from build123d import *

# Parameters (mm, degrees)
F1_DEPTH = 63.5
F0_W     = 19.703557321
F0_H     = 14.5021951942
F2_DEPTH = 25.4
F3_DEPTH = 7.9375
F5_R     = 6.35


with BuildPart() as f1:
    # F0 (on Front) → F1 (new body, symmetric)
    with BuildSketch(Plane.XZ):
        Polygon((-41.275, 9.525), (-41.275, -9.525), (41.275, -9.525), (41.275, 9.525), (22.225, 9.525), align=None)
    extrude(amount=F1_DEPTH, both=True)

    # F0 (on Front) → F2 (join, symmetric)
    with BuildSketch(Plane.XZ):
        with BuildLine():
            Line((22.225, 9.525), (41.275, 9.525))
            Line((41.275, 9.525), (41.275, 31.7500035657))
            ThreePointArc((41.275, 31.7500035657), (44.6674064176, 39.9399971481), (52.8574, 43.3324035657))
            Line((52.8574, 43.3324035657), (64.774647217, 43.3324035657))
            Line((64.774647217, 43.3324035657), (64.774647217, 57.8345987598))
            Line((64.774647217, 57.8345987598), (84.478204538, 57.8345987598))
            Line((84.478204538, 57.8345987598), (84.478204538, 62.3824035657))
            Line((84.478204538, 62.3824035657), (52.8574, 62.3824035657))
            ThreePointArc((52.8574, 62.3824035657), (31.197022236, 53.4103813297), (22.225, 31.7500035657))
            Line((22.225, 31.7500035657), (22.225, 9.525))
        make_face()
        with Locations((74.6264258775, 50.5835011627)):
            Rectangle(F0_W, F0_H)
    extrude(amount=F2_DEPTH, both=True)

    # F0 (on Front) → F3 (join, symmetric)
    with BuildSketch(Plane.XZ):
        with BuildLine():
            add(Edge.make_bspline(
                [(-41.275, 9.525), (-35.4120545089, 64.6761879325), (31.4773879945, 74.0210413933), (84.478204538, 62.3824035657)],
                knots=[0, 0, 0, 0, 136.4103132585, 136.4103132585, 136.4103132585, 136.4103132585], degree=3))
            Line((-41.275, 9.525), (22.225, 9.525))
            Line((22.225, 9.525), (22.225, 31.7500035657))
            ThreePointArc((22.225, 31.7500035657), (31.197022236, 53.4103813297), (52.8574, 62.3824035657))
            Line((52.8574, 62.3824035657), (84.478204538, 62.3824035657))
        make_face()
    extrude(amount=F3_DEPTH, both=True)

    # F0 (on Front) → F4 (revolve)
    with BuildSketch(Plane.XZ):
        Polygon((115.574647217, 57.8345987598), (84.478204538, 57.8345987598), (84.478204538, 43.3324035657), (84.478204538, 32.6885987598), (115.574647217, 32.6885987598), align=None)
    revolve(axis=Axis((84.478204538, 0, 47.5355011627), (0, 0, -1)))

    # F5
    f5_edges = [f1.edges().sort_by_distance(p)[0] for p in [
        (41.275, -63.5, 0),
        (-41.275, -63.5, 0),
        (-41.275, 63.5, 0),
        (41.275, 63.5, 0),
    ]]
    fillet(f5_edges, radius=F5_R)


solid = f1.part
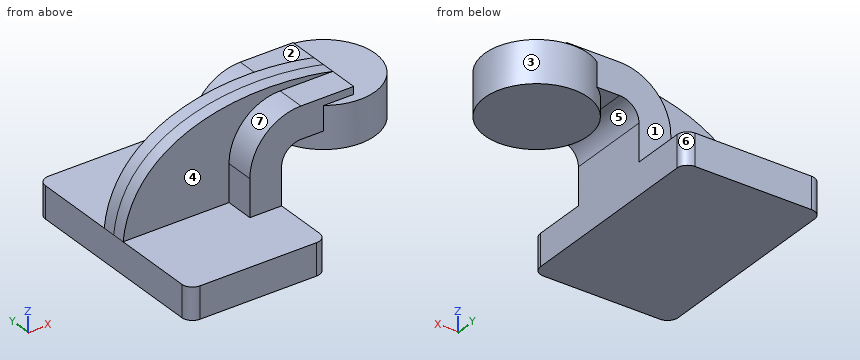
Design review of the part built by this model. Coordinates are the model's own, in mm. Face numbers are marked on the shaded views. A direction names the side the tool comes from. Give positions to 0.01 mm unless a question says otherwise; leave off trailing zeros. Order: outer loops, then holes, each group sorted by start corner. A loop starts at its lowest first (then second) coordinate and runs counter-clockwise, first axis right, second up.
1. Add section B-B, the plane y = 36.5. State the section outline as (x, z) points (3 decimals).
Solution:
outline: (-41.275, -9.525) - (41.275, -9.525) - (41.275, 9.525) - (-41.275, 9.525) - close
2. For pin 1 Ø5 at (y, z) = (-17, 40.5) entering from +X; pin 2 Ø4 at (x, y) = (6, -14) entering from +Z (3 decimals); pin 3 Ø4 at (x, y) = (63, 2.5) entering from -Z, all flat-tipped, find the tip position at first contact; note any pin that passes through.
Solution:
pin 1: stops at x = 111.99
pin 2: stops at z = 9.525
pin 3: stops at z = 32.69
3. To check wall thickness, follow L1, parallel to Z at x = 19, y = 35 (3 decimals); L2, parallel to Z at x = 81, y = -27; L3, parallel to X at y = -16, z = 1.5 (3 decimals). State the ranges of each line that lie inside material, in increasing order.
Solution:
L1: z = -9.525 to 9.525
L2: z = 32.69 to 57.83
L3: x = -41.275 to 41.275
4. Tool access review of the marked faces 1, 2, 3 and 4: name each direction out of +Z, -Z, +X, -X, +Y, -Y from which nothing blocks a thin tool from reaching the whole face with its end or side.
Solution:
face 1: +Z, -X, +Y
face 2: +Z, +X, -X, +Y
face 3: -Z
face 4: +Z, -X, -Y
5. Add section A-A, the plane y = 19. State the section outline as (x, z) points (3 decimals), then the cut area to 3 significant figures.
Solution:
outline: (-41.275, -9.525) - (41.275, -9.525) - (41.275, 31.75) arc R11.582 cw to (52.857, 43.332) - (59.861, 43.332) - (59.861, 32.689) - (109.095, 32.689) - (109.095, 57.835) - (84.478, 57.835) - (84.478, 62.382) - (52.857, 62.382) arc R30.632 ccw to (22.225, 31.75) - (22.225, 9.525) - (-41.275, 9.525) - close
area: 4,110 mm2
6. Mouldability with a two-part tool opening along X and no side actions: class the marked faces 5, 6 and 7 as +X half, -X half, draft (parallel to the pull), parting line (faces both ways), or undercut.
Solution:
face 5: undercut
face 6: +X half
face 7: -X half
